Job drawing, mm, ordinate dimensions from the low corner. One solid piece. Give positions to 0.01 mm unless a question says otherwise; leave off trailing zeros. Loops run counter-clockwise (first coordinate to the right, second up) from the corner with the lowest first, then second, coordinate; pieces in that order, holes last. Notation, with made-up numbers: M 87.5,87 L 97.5,87 A18 cw 97.5,96 Z; hole C 60.5,-22 d4. An arc over 180 degrees is marked long. Answer in a Markdown table with one row per item.
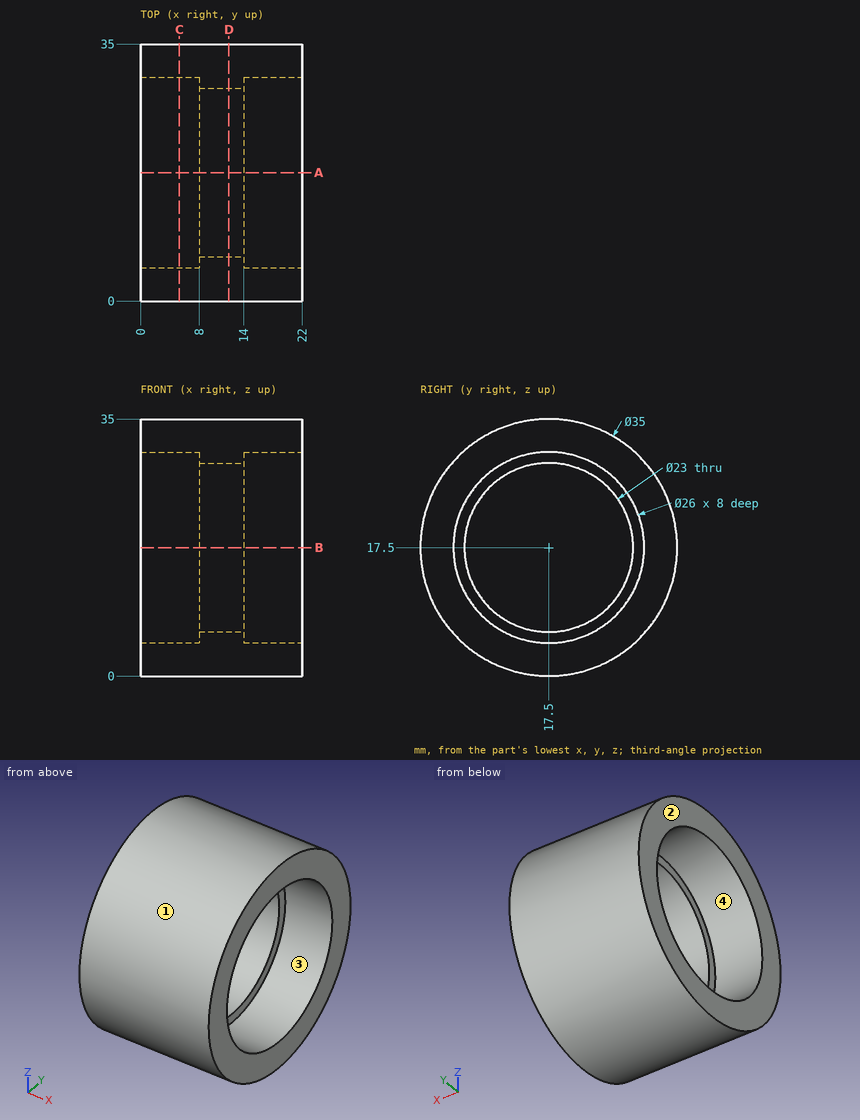
(1) Saw through at A-A (y = 17.5). Write the cut outline in (x, z), plus the area to 3 significant figures.
Recorded:
| item | result |
|---|---|
| outline | M 0,0 L 22,0 L 22,4.5 L 14,4.5 L 14,6 L 8,6 L 8,4.5 L 0,4.5 Z; M 0,30.5 L 8,30.5 L 8,29 L 14,29 L 14,30.5 L 22,30.5 L 22,35 L 0,35 Z |
| area | 216 mm^2 |
(2) Saw through at D-D (x = 12). Write the cut outline in (y, z).
Recorded:
| item | result |
|---|---|
| outline | C 17.5,17.5 d35; hole C 17.5,17.5 d23 |
(3) Drill centre lines: line 1 along Z through (x, y) = (10.45, 17.5); line 2 along Z through (x, y) = (18.5, 17.5); line 3 along Y through (x, z) = (11.75, 11). Where is each one in solid material? Low to high.
Recorded:
| item | result |
|---|---|
| line 1 | z = 0 to 6, 29 to 35 |
| line 2 | z = 0 to 4.5, 30.5 to 35 |
| line 3 | y = 1.25 to 8.01, 26.99 to 33.75 |
(4) Pin check, flat tips, straight feed: pin 1 Ø5 at (x, y) = (18.5, 10.5) entering from +Z; pin 2 Ø1.5 at (x, y) = (4.5, 16.5) entering from +Z; pin 3 Ø1 at (y, z) = (25, 9.5) entering from +X; pin 4 Ø4 at (x, y) = (19, 11.5) entering from +Z. Stop position of each tip, or through.
Recorded:
| item | result |
|---|---|
| pin 1 | stops at z = 34.41 |
| pin 2 | stops at z = 35 |
| pin 3 | passes through |
| pin 4 | stops at z = 34.54 |
(5) Saw through at C-C (x = 5.25). Write the cut outline in (y, z).
Recorded:
| item | result |
|---|---|
| outline | C 17.5,17.5 d35; hole C 17.5,17.5 d26 |
(6) Pull direction Y, two halves, no side cores. Call the marked faces 1, 2, 3 and 4: +Y half, -Y half, draft (parallel to the pull), parting line (faces both ways), or undercut.
Recorded:
| item | result |
|---|---|
| face 1 | parting line |
| face 2 | draft |
| face 3 | undercut |
| face 4 | undercut |
